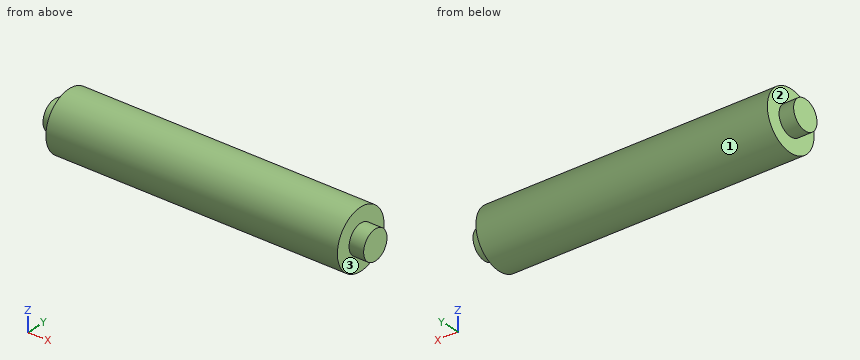
from build123d import *

# Parameters (mm, degrees)
SKETCH1_R           = 76.2
BOSS_EXTRUDE1_DEPTH = 76.2
SKETCH2_R           = 152.4
BOSS_EXTRUDE2_DEPTH = 1524
SKETCH3_R           = 76.2
BOSS_EXTRUDE3_DEPTH = 76.2


with BuildPart() as part:
    # Sketch1 → Boss-Extrude1 (new body)
    with BuildSketch(Plane(origin=(0, 0, 0), x_dir=(0, 0, -1), z_dir=(1, 0, 0))):
        Circle(SKETCH1_R)
    extrude(amount=BOSS_EXTRUDE1_DEPTH)

    # Sketch2 → Boss-Extrude2 (add)
    with BuildSketch(Plane(origin=(76.2, 0, 0), x_dir=(0, 0, -1), z_dir=(1, 0, 0))):
        Circle(SKETCH2_R)
    extrude(amount=BOSS_EXTRUDE2_DEPTH)

    # Sketch3 → Boss-Extrude3 (add)
    with BuildSketch(Plane(origin=(1600.2, 0, 0), x_dir=(0, 0, -1), z_dir=(1, 0, 0))):
        Circle(SKETCH3_R)
    extrude(amount=BOSS_EXTRUDE3_DEPTH)


solid = part.part
Build history of the part. All positions in model axes, mm. Face numbers are marked on the shaded views. A direction names the side the tool comes from. Coordinates: 2 decimals unless noted, no trailing zeros. Order: outer loops, then holes, each group sorted by start corner. A loop starts at its lowest first (then second) coordinate and runs counter-clockwise, first axis right, second up. Notation, with made-up numbers: (34, 16.5) - (73, 16.5) arc R10 ccw to (73, 23.5) - close; hole circle Ø8 at (-38.5, 19.25). An arc over 180 degrees is marked (long way). Put each result on its own line as item: value.
1. Drop flat-ended pins along their axis: P1, Ø6, axis at x = 1459, y = 72, coming from the +Z side; P2, Ø1, axis at x = 377, z = 46.5, coming from the +Y side; P3, Ø2, axis at x = 1328, z = -61, coming from the -Y side. Give the stop position or say it passes through.
Answer sheet:
P1: stops at z = 135.89
P2: stops at y = 145.29
P3: stops at y = -140.09
2. Saw through at A-A (y = 0). Write the cut outline in (x, z), and give its area (3 significant figures).
Answer sheet:
outline: (0, -76.2) - (76.2, -76.2) - (76.2, -152.4) - (1600.2, -152.4) - (1600.2, -76.2) - (1676.4, -76.2) - (1676.4, 76.2) - (1600.2, 76.2) - (1600.2, 152.4) - (76.2, 152.4) - (76.2, 76.2) - (0, 76.2) - close
area: 488,000 mm^2
3. Tool access for the marked faces 1, 2 and 3: list every direction of +Z, -Z, +X, -X, +Y, -Y with a clear straight run to the whole face (end or side of a thin tool).
Answer sheet:
face 1: +X, -X
face 2: -X
face 3: +X
4. Probe line 1 along X through (y, z) = (133, 34); line 2 along Y through (x, z) = (1130, 10); line 3 along Y through (x, z) = (613, -8). List the from-to ranges inside material, lowest first. Write a range as [from, to].
Answer sheet:
line 1: x = [76.2, 1600.2]
line 2: y = [-152.07, 152.07]
line 3: y = [-152.19, 152.19]
5. Saw through at D-D (z = -103). Write the cut outline in (x, y).
Answer sheet:
outline: (76.2, -112.32) - (1600.2, -112.32) - (1600.2, 112.32) - (76.2, 112.32) - close
6. Saw through at C-C (x = 345). Write the cut outline in (y, z).
Answer sheet:
outline: circle Ø304.8 at (0, 0)
